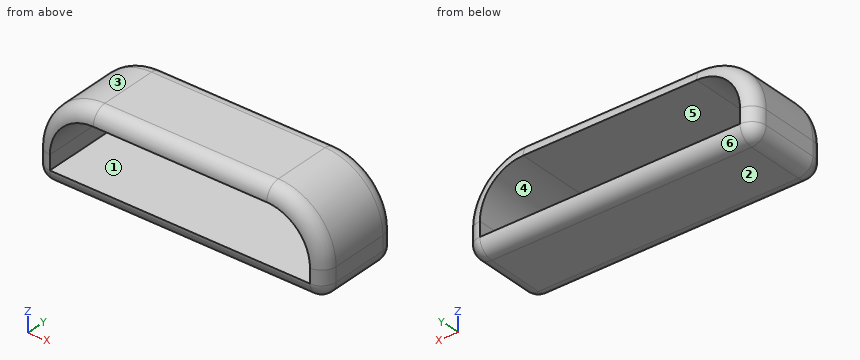
```python
from build123d import *

# Parameters (mm, degrees)
F1_DEPTH = 15
F2_R     = 2.5
F4_DEPTH = 15.001


with BuildPart() as f1:
    # F0 (on Front) → F1 (new body)
    with BuildSketch(Plane.XZ):
        with BuildLine():
            Line((-34.4305347418, 15), (-64.4305347418, 15))
            ThreePointArc((-64.4305347418, 15), (-71.5016025537, 12.0710678119), (-74.4305347418, 5))
            Line((-74.4305347418, 5), (-24.4305347418, 5))
            ThreePointArc((-24.4305347418, 5), (-27.3594669299, 12.0710678119), (-34.4305347418, 15))
        make_face()
        with BuildLine():
            Line((-24.4305347418, 5), (-74.4305347418, 5))
            Line((-74.4305347418, 5), (-74.4305347418, 2.5))
            ThreePointArc((-74.4305347418, 2.5), (-73.6983016948, 0.732233047), (-71.9305347418, 0))
            Line((-71.9305347418, 0), (-26.9305347418, 0))
            ThreePointArc((-26.9305347418, 0), (-25.1627677888, 0.732233047), (-24.4305347418, 2.5))
            Line((-24.4305347418, 2.5), (-24.4305347418, 5))
        make_face()
    extrude(amount=F1_DEPTH)

    # F2
    f2_edges = [f1.edges().sort_by_distance(p)[0] for p in [
        (-64.430535, -7.5, 15),
        (-74.430535, -7.5, 5),
        (-71.501603, 0, 12.071068),
        (-71.501603, -15, 12.071068),
    ]]
    fillet(f2_edges, radius=F2_R)

    # F3 (on face) → F4 (cut, through all)
    with BuildSketch(Plane.XZ.offset(15)):
        with BuildLine():
            Line((-34.4305347418, 12.5), (-64.4305347418, 12.5))
            ThreePointArc((-64.4305347418, 12.5), (-69.7338356007, 10.3033008589), (-71.9305347418, 5))
            Line((-71.9305347418, 5), (-71.9305347418, 2.5))
            Line((-71.9305347418, 2.5), (-26.9305347418, 2.5))
            Line((-26.9305347418, 2.5), (-26.9305347418, 5))
            ThreePointArc((-26.9305347418, 5), (-29.1272338829, 10.3033008589), (-34.4305347418, 12.5))
        make_face()
    extrude(amount=-F4_DEPTH, mode=Mode.SUBTRACT)


solid = f1.part
```
Model file for the job. Use its own axes, mm. Face numbers are marked on the shaded views. A direction names the side the tool comes from. Round coordinates to 2 decimals unless told otherwise and drop trailing zeros. Order: outer loops, then holes, each group sorted by start corner. A loop starts at its lowest first (then second) coordinate and runs counter-clockwise, first axis right, second up. Notation, with made-up numbers: M 17,13.5 L 42,13.5 A19 ccw 42,36.5 Z; hole C 74.5,89 d9. An arc over 180 degrees is marked long. Use CSV: the item, a comma, the result in double quotes.
Item 1: Pull direction Z, two halves, no side cores. Call the marked faces 1, 2, 3 and 4: released by +Z, released by -Z, zero draft, split by the parting line, or undercut.
Worked answers:
face 1,"undercut"
face 2,"released by -Z"
face 3,"released by +Z"
face 4,"undercut"
Item 2: Which spindle directions (+Z, -Z, +X, -X, +Y, -Y) get a long thin tool onto all of the face, cutting with end or side? Do the marked faces 5 and 6. Say none if no direction does.
Worked answers:
face 5,"+Y, -Y"
face 6,"-Z, +X, -X, +Y"
Item 3: Probe probe 1 along Z at (x, y) = (-45.5, -9.25); probe 2 along X at (y, z) = (-6.5, 4.75); probe 3 along X at (y, z) = (-4.5, 11). List the from-to ranges inside material, lowest first.
Worked answers:
probe 1,"0 to 2.5, 12.5 to 15"
probe 2,"-74.43 to -71.93, -26.93 to -24.43"
probe 3,"-72.43 to -68.93, -29.93 to -26.43"
Item 4: Saw through at B-B (y = -9.5). List the corners of the cut face in (x, z), plus the area to 3 significant figures.
Worked answers:
outline,"M -74.43,2.5 A2.5 ccw -71.93,0 L -26.93,0 A2.5 ccw -24.43,2.5 L -24.43,5 A10 ccw -34.43,15 L -64.43,15 A10 ccw -74.43,5 Z; hole M -71.93,2.5 L -26.93,2.5 L -26.93,5 A7.5 ccw -34.43,12.5 L -64.43,12.5 A7.5 ccw -71.93,5 Z"
area,"279 mm²"
Item 5: Pin check, flat tips, straight feed: pin 1 (6 mm diameter, centred on x = -30, z = 4, fed in from +Y); pin 2 (1 mm diameter, centred on y = -5.5, z = 11, fed in from -X); pin 3 (6 mm diameter, centred on y = -7.5, z = 9, fed in from +X). Stop position of each tip, or through.
Worked answers:
pin 1,"y = 0"
pin 2,"x = -72.78"
pin 3,"x = -24.48"
Item 6: Saw through at C-C (y = -1.5). List the corners of the cut face in (x, z), plus the area to 3 significant figures.
Worked answers:
outline,"M -74.22,2.5 A2.29 ccw -71.93,0.21 L -26.93,0.21 A2.29 ccw -24.64,2.5 L -24.64,5 A9.79 ccw -34.43,14.79 L -64.43,14.79 A9.79 ccw -74.22,5 Z; hole M -71.93,2.5 L -26.93,2.5 L -26.93,5 A7.5 ccw -34.43,12.5 L -64.43,12.5 A7.5 ccw -71.93,5 Z"
area,"254 mm²"
Item 7: Saw through at A-A (x = -35.5). List the corners of the cut face in (y, z).
Worked answers:
outline,"M -15,2.5 A2.5 ccw -12.5,0 L -2.5,0 A2.5 ccw 0,2.5 Z; M -15,12.5 L 0,12.5 A2.5 ccw -2.5,15 L -12.5,15 A2.5 ccw Z"
